```python
from build123d import *

# Parameters (mm, degrees)
F1_DEPTH = 80
F2_SIZE2 = 60
F2_SIZE  = 25
F3_SIZE2 = 5
F3_SIZE  = 47
F4_SIZE  = 10
F5_SIZE2 = 20
F5_SIZE  = 15
F6_SIZE  = 12


with BuildPart() as f1:
    # F0 (on Front) → F1 (new body)
    with BuildSketch(Plane.XZ):
        Polygon((-124.2189471151, -0.7847668109), (-145.6560869584, -45.9560966047), (154.3439130416, -45.9560966047), (134.6452535731, 0), (62.5519627112, 20.6774614667), align=None)
    extrude(amount=-F1_DEPTH)

    # F2
    f2_edges = [f1.edges().sort_by_distance(p)[0] for p in [
        (-30.833492, 80, 9.946347),
        (98.598608, 80, 10.338731),
        (144.494583, 80, -22.978048),
        (-134.937517, 80, -23.370432),
    ]]
    f2_side = f1.faces().sort_by_distance((8.549856, 80, -18.412725))[0]
    chamfer(f2_edges, length=F2_SIZE, length2=F2_SIZE2, reference=f2_side)

    # F3
    f3_edges = [f1.edges().sort_by_distance(p)[0] for p in [
        (-30.833492, 0, 9.946347),
        (-134.937517, 0, -23.370432),
        (98.598608, 0, 10.338731),
        (144.494583, 0, -22.978048),
    ]]
    f3_side = f1.faces().sort_by_distance((8.549856, 0, -18.412725))[0]
    chamfer(f3_edges, length=F3_SIZE, length2=F3_SIZE2, reference=f3_side)

    # F4
    f4_edges = [f1.edges().sort_by_distance(p)[0] for p in [
        (88.397911, 80, -12.743521),
    ]]
    chamfer(f4_edges, length=F4_SIZE)

    # F5
    f5_edges = [f1.edges().sort_by_distance(p)[0] for p in [
        (-36.512691, 80, -15.870779),
    ]]
    f5_side = f1.faces().sort_by_distance((-28.16235, 49.160168, -1.976733))[0]
    chamfer(f5_edges, length=F5_SIZE, length2=F5_SIZE2, reference=f5_side)

    # F6
    f6_edges = [f1.edges().sort_by_distance(p)[0] for p in [
        (-117.819987, 43.076923, -9.72811),
    ]]
    chamfer(f6_edges, length=F6_SIZE)


solid = f1.part
```
Geometry: final body of the model. Coordinates: model frame, mm. Coordinates: 2 decimals unless noted, no trailing zeros. Loops run counter-clockwise (first coordinate to the right, second up) from the corner with the lowest first, then second, coordinate; pieces in that order, holes last. Notation, with made-up numbers: (26, 39.25) -> (69, 39.25) arc R16 cw to (69, 59.25) -> close; hole circle Ø4 at (46, 43.25). An arc over 180 degrees is marked (long way). Use a Markdown table: item, result. Add a question column.
(1) Section query B-B, the plane x = 74.5. Return loops of the section in (y, z).
(2) Pin query (flat end, axial travel): pin 1 Ø3 at (y, z) = (47.5, -17.5) entering from -X; pin 2 Ø5 at (x, y) = (60.5, 34) entering from +Z; pin 3 Ø8 at (x, z) = (-73.5, -6) entering from -Y. Return the tip coordinate at first contact, or that it passes through.
(3) Line query: line 1 along Z through (x, y) = (62, 12.5); line 2 along X through (y, z) = (11, -8); line 3 along Z through (x, y) = (-44.5, 8.5). Output: solid intervals per line, ascending.
(4) Section query A-A, the plane z = -30. Return loops of the section in (x, y), plus the area to 3 significant figures.
(5) Section query C-C, the plane y = 48.5. Return loops of the section in (x, z), plus the area to 3 significant figures.
(6) Section query D-D, the plane x = -2. Return loops of the section in (y, z).
Answer:
| question | item | result |
|---|---|---|
| 1 | outline | (0, -45.96) -> (80, -45.96) -> (80, -23.25) -> (69.94, -4.4) -> (20, 17.25) -> (5, 17.25) -> (0, -31.64) -> close |
| 2 | pin 1 | stops at x = -117.26 |
| 2 | pin 2 | stops at z = 15.66 |
| 2 | pin 3 | stops at y = 3.41 |
| 3 | line 1 | z = -45.96 to 20.61 |
| 3 | line 2 | x = -127.64 to 138.07 |
| 3 | line 3 | z = -45.96 to 8.38 |
| 4 | outline | (-138.08, 5) -> (-103.32, 1.66) -> (33.24, 0) -> (68.77, 0) -> (108.2, 1.16) -> (147.5, 5) -> (147.5, 20) -> (121.03, 78.39) -> (112.29, 80) -> (15.72, 80) -> (-112.1, 72.16) -> (-116.51, 66.78) -> (-138.08, 20) -> close |
| 4 | area | 20,300 mm^2 |
| 5 | outline | (-132.51, -45.96) -> (141.42, -45.96) -> (125.95, -9.86) -> (61.55, 8.61) -> (-104.13, -10.43) -> (-121.58, -22.92) -> close |
| 5 | area | 11,300 mm^2 |
| 6 | outline | (0, -45.96) -> (80, -45.96) -> (80, -32.04) -> (66.15, -6.1) -> (20, 13.26) -> (5, 13.26) -> (0, -34.05) -> close |
